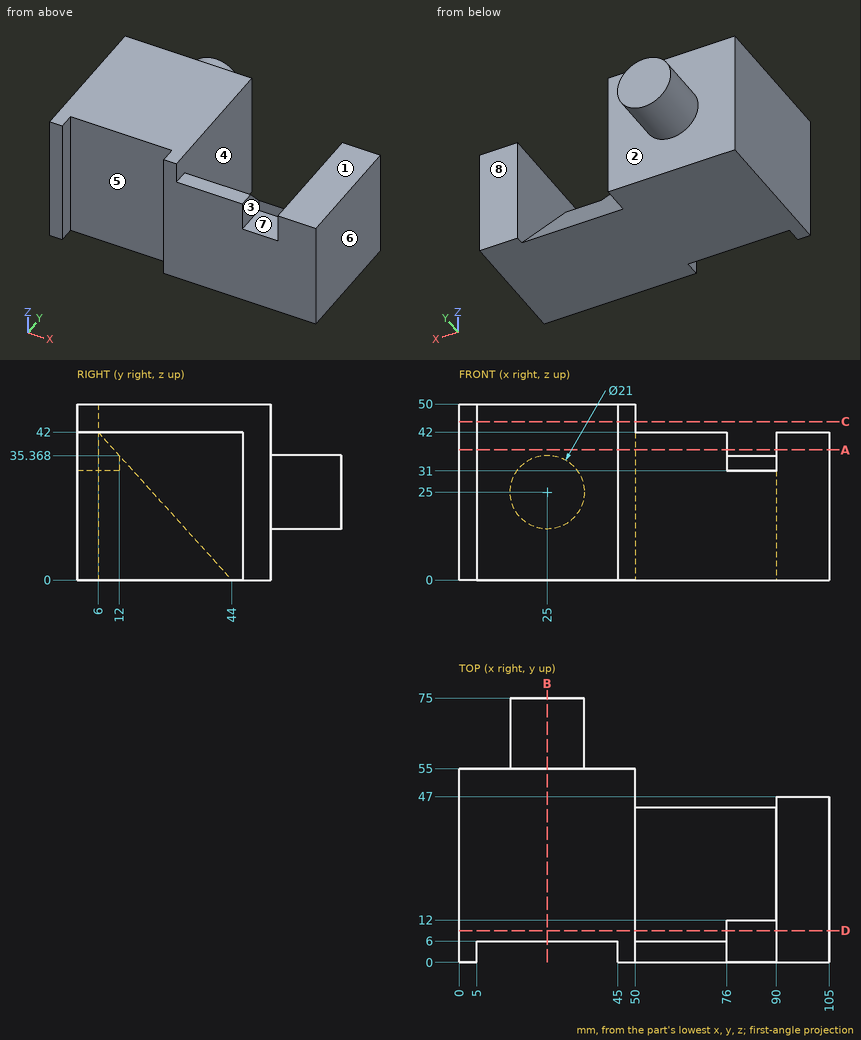
Geometry check sheet. Reference: drawing and pictorial views, mm from the part's lowest x, y, z. A direction names the side the tool comes from. Coordinates: 2 decimals unless noted, no trailing zeros. Write each loop counter-clockwise with the first axis right and the second up, starting at its lowest first coordinate (ties: lowest second). Pieces come first, ordered by that corner, then holes.
Item 1: Mould release check, pull along X, two halves, no side actions. Record for the marked faces 6, 7 and 8: released by +X, released by -X, zero draft, split by the parting line, or undercut.
Numbers:
face 6: released by +X
face 7: undercut
face 8: zero draft
Item 2: Cross-section at B-B on x = 25. Record the boundary of the cut face in (y, z), then the cut area to 3 significant figures.
Numbers:
outline: (6, 0) - (55, 0) - (55, 14.5) - (75, 14.5) - (75, 35.5) - (55, 35.5) - (55, 50) - (6, 50) - close
area: 2,870 mm2
Item 3: Scan lines: probe 1 along X at (y, z) = (18.5, 31); probe 2 along Y at (x, z) = (25.5, 22.5); probe 3 along Y at (x, z) = (9, 36). Record each from-to range of solid material in increasing order.
Numbers:
probe 1: x = 0 to 50, 90 to 105
probe 2: y = 6 to 75
probe 3: y = 6 to 55
Item 4: Access from +Z, -Z, +X, -X, +Y, -Y to the whole of each face (thin tool, end or side, straight path). Record for the marked faces 1, 2, 3, 4 and 5.
Numbers:
face 1: +Z, +X, +Y, -Y
face 2: +Y
face 3: +Z, -Y
face 4: +Z, +Y
face 5: +Z, -Z, -Y
Item 5: Depth check by flat-ended pin: pin 1 Ø16.5 at (x, y) = (99, 15.5) entering from +Z; pin 2 Ø1.3 at (x, z) = (83, 33) entering from -Y; pin 3 Ø1.5 at (x, z) = (60.5, 13.5) entering from +Y (1 decimal). Enter the tip coordinate at first touch or a pass-through.
Numbers:
pin 1: stops at z = 42
pin 2: stops at y = 12
pin 3: stops at y = 32.5
Item 6: Cross-section at A-A on z = 37. Record the boundary of the cut face in (x, y), then the cut area to 3 significant figures.
Numbers:
outline: (0, 0) - (5, 0) - (5, 6) - (45, 6) - (45, 0) - (76, 0) - (76, 10.52) - (50, 10.52) - (50, 55) - (0, 55) - close; (90, 0) - (105, 0) - (105, 47) - (90, 47) - close
area: 3,490 mm2
Item 7: Cross-section at C-C on z = 45. Record the boundary of the cut face in (x, y).
Numbers:
outline: (0, 0) - (5, 0) - (5, 6) - (45, 6) - (45, 0) - (50, 0) - (50, 55) - (0, 55) - close
Item 8: Cross-section at D-D on y = 9. Record the boundary of the cut face in (x, z) (1 decimal).
Numbers:
outline: (0, 0) - (105, 0) - (105, 42) - (90, 42) - (90, 31) - (76, 31) - (76, 38.7) - (50, 38.7) - (50, 50) - (0, 50) - close
